```python
from build123d import *

# Parameters (mm, degrees)
SKETCH1_W           = 45
SKETCH1_H           = 45
SKETCH1_R           = 2.6
BOSS_EXTRUDE1_DEPTH = 7.5
SKETCH2_R           = 8.1
CUT_EXTRUDE1_DEPTH  = 6
CUT_EXTRUDE4_START  = -6
SKETCH5_R           = 8.1
CUT_EXTRUDE4_DEPTH  = 6
SKETCH7_W           = 37
SKETCH7_H           = 7
BOSS_EXTRUDE2_DEPTH = 10
CUT_EXTRUDE6_START  = 2
CUT_EXTRUDE6_DEPTH  = 3.6
SKETCH8_R           = 2.1
CUT_EXTRUDE7_DEPTH  = 43.278836313
SKETCH9_W           = 3
SKETCH9_H           = 7
BOSS_EXTRUDE3_DEPTH = 10
SKETCH10_W          = 7
SKETCH10_H          = 7
BOSS_EXTRUDE4_DEPTH = 2
CHAMFER2_SIZE2      = 7
CHAMFER2_SIZE       = 2
CHAMFER3_SIZE2      = 7
CHAMFER3_SIZE       = 2


with BuildPart() as part:
    # Sketch1 → Boss-Extrude1 (new, symmetric)
    with BuildSketch(Plane.XY):
        Rectangle(SKETCH1_W, SKETCH1_H)
        Circle(SKETCH1_R, mode=Mode.SUBTRACT)
    extrude(amount=BOSS_EXTRUDE1_DEPTH, both=True)

    # Sketch2 → Cut-Extrude1 (cut)
    with BuildSketch(Plane.XY.offset(7.5)):
        Circle(SKETCH2_R)
    extrude(amount=-CUT_EXTRUDE1_DEPTH, mode=Mode.SUBTRACT)

    # Sketch5 → Cut-Extrude4 (cut)
    with BuildSketch(Plane(origin=(0, 0, -7.5), x_dir=(-1, 0, 0), z_dir=(0, 0, -1)).offset(CUT_EXTRUDE4_START)):
        with Locations(Location((0, 0, 0), (0, 0, 180))):
            Circle(SKETCH5_R)
    extrude(amount=CUT_EXTRUDE4_DEPTH, mode=Mode.SUBTRACT)

    # Sketch7 → Boss-Extrude2 (add)
    with BuildSketch(Plane.XZ.offset(22.5)):
        Rectangle(SKETCH7_W, SKETCH7_H)
    extrude(amount=BOSS_EXTRUDE2_DEPTH)

    # Sketch6 → Cut-Extrude6 (cut)
    with BuildSketch(Plane.XY.offset(-7.5).offset(CUT_EXTRUDE6_START)):
        Polygon((19.2, 17.636195996), (15.5, 19.772391992), (11.8, 17.636195996), (11.8, 13.363804004), (15.5, 11.227608008), (19.2, 13.363804004), align=None)
        Polygon((-11.8, 17.636195996), (-15.5, 19.772391992), (-19.2, 17.636195996), (-19.2, 13.363804004), (-15.5, 11.227608008), (-11.8, 13.363804004), align=None)
        Polygon((19.2, -13.363804004), (15.5, -11.227608008), (11.8, -13.363804004), (11.8, -17.636195996), (15.5, -19.772391992), (19.2, -17.636195996), align=None)
        Polygon((-11.8, -13.363804004), (-15.5, -11.227608008), (-19.2, -13.363804004), (-19.2, -17.636195996), (-15.5, -19.772391992), (-11.8, -17.636195996), align=None)
    extrude(amount=CUT_EXTRUDE6_DEPTH, mode=Mode.SUBTRACT)

    # Sketch8 → Cut-Extrude7 (cut, through all)
    with BuildSketch(Plane(origin=(0, 0, -7.5), x_dir=(-1, 0, 0), z_dir=(0, 0, -1))):
        with Locations((-15.5, 15.5)):
            Circle(SKETCH8_R)
        with Locations((15.5, 15.5)):
            Circle(SKETCH8_R)
        with Locations((15.5, -15.5)):
            Circle(SKETCH8_R)
        with Locations((-15.5, -15.5)):
            Circle(SKETCH8_R)
    extrude(amount=-CUT_EXTRUDE7_DEPTH, mode=Mode.SUBTRACT)

    # Sketch9 → Boss-Extrude3 (add)
    with BuildSketch(Plane.XZ.offset(32.5)):
        with Locations((-17, 0)):
            Rectangle(SKETCH9_W, SKETCH9_H)
        with Locations((17, 0)):
            Rectangle(SKETCH9_W, SKETCH9_H)
    extrude(amount=BOSS_EXTRUDE3_DEPTH)

    # Sketch10 → Boss-Extrude4 (add)
    with BuildSketch(Plane.ZY.offset(18.5)):
        with Locations((0, -39)):
            Rectangle(SKETCH10_W, SKETCH10_H)
    boss_extrude4 = extrude(amount=BOSS_EXTRUDE4_DEPTH)

    # Mirror1: Boss-Extrude4 across plane
    add(boss_extrude4.mirror(Plane(origin=(0, 0, 0), x_dir=(0, 0, 1), z_dir=(1, 0, 0))))

    # Chamfer2
    chamfer2_edges = [part.edges().sort_by_distance(p)[0] for p in [
        (-20.5, -42.5, 0),
    ]]
    chamfer2_side = [part.faces().sort_by_distance(p)[0] for p in [
        (-20.46, -42.5, 0),
    ]]
    chamfer(chamfer2_edges, length=CHAMFER2_SIZE - 0.0001, length2=CHAMFER2_SIZE2 - 0.0001, reference=chamfer2_side[0])  # a hair under: the kernel refuses the full size

    # Chamfer3
    chamfer3_edges = [part.edges().sort_by_distance(p)[0] for p in [
        (20.5, -42.5, 0),
    ]]
    chamfer3_side = [part.faces().sort_by_distance(p)[0] for p in [
        (20.46, -42.5, 0),
    ]]
    chamfer(chamfer3_edges, length=CHAMFER3_SIZE - 0.0001, length2=CHAMFER3_SIZE2 - 0.0001, reference=chamfer3_side[0])  # a hair under: the kernel refuses the full size


solid = part.part
```
Geometry: final body of the model. Coordinates: model frame, mm. A direction names the side the tool comes from. Round coordinates to 2 decimals unless told otherwise and drop trailing zeros. Order: outer loops, then holes, each group sorted by start corner. A loop starts at its lowest first (then second) coordinate and runs counter-clockwise, first axis right, second up. Notation, with made-up numbers: (49.25, 31) -> (77.25, 31) arc R12 ccw to (77.25, 53) -> close; hole circle Ø2 at (43.5, 18.25). An arc over 180 degrees is marked (long way). Write each question's results on one line, items separated by ' | '.
Q1. Section query C-C (z = 0.75). Count the separate pieces of the cut face and the enclosed holes in it, and give its area (3 significant figures).
Response values:
separate pieces: 1 | enclosed holes: 5 | area: 2,390 mm²
Q2. Pin query (flat end, axial travel): pin 1 Ø8 at (x, y) = (0, -0.5) entering from +Z; pin 2 Ø3 at (y, z) = (-25, -2.5) entering from +X; pin 3 Ø3 at (x, y) = (0, 0) entering from -Z; pin 4 Ø7.5 at (y, z) = (-28.5, -1.5) entering from -X. Return the tip coordinate at first contact, or that it passes through.
Response values:
pin 1: z = 1.5 | pin 2: x = 18.5 | pin 3: through | pin 4: x = -18.5
Q3. Access query for faces 4 (the face through (-1.756, -7.907, 4.542)), 5 (the face through (0, -32.5, 0)), 6 (the face through (13.68, -12.28, -3.73)). Directions: +Z, -Z, +X, -X, +Y, -Y. A direction counts if a zero-diameter tool reaches every point of the face in a straight line with its end or side. Return the directions, or none.
Response values:
face 4: +Z | face 5: +Z, -Z, -Y | face 6: none
Q4. Ray query, line 1 along X through (y, z) = (17.5, -3); line 2 along Z through (x, y) = (18.5, -14.5). Return the intervals inside material, ascending.
Response values:
line 1: -22.5 to -19.2, -11.8 to 11.8, 19.2 to 22.5 | line 2: -7.5 to -5.5, -1.9 to 7.5
Q5. Pull-direction query (Z, two-part tool) for faces 1 (the face through (0, 10, 7.5)), 2 (the face through (17.376, -12.311, -3.725)), 3 (the face through (-15.227, -13.418, 2.734)); classes: released by +Z, released by -Z, zero draft, split by the parting line, or undercut.
Response values:
face 1: released by +Z | face 2: undercut | face 3: zero draft
Q6. Section query D-D (y = 0). Output: boundary loops of the cut face in (x, z).
Response values:
outline: (-22.5, -7.5) -> (-8.1, -7.5) -> (-8.1, -1.5) -> (-2.6, -1.5) -> (-2.6, 1.5) -> (-8.1, 1.5) -> (-8.1, 7.5) -> (-22.5, 7.5) -> close; (2.6, -1.5) -> (8.1, -1.5) -> (8.1, -7.5) -> (22.5, -7.5) -> (22.5, 7.5) -> (8.1, 7.5) -> (8.1, 1.5) -> (2.6, 1.5) -> close
Q7. Section query A-A (x = 0). Output: boundary loops of the cut face in (y, z), and give its area (3 significant figures).
Response values:
outline: (-32.5, -3.5) -> (-22.5, -3.5) -> (-22.5, -7.5) -> (-8.1, -7.5) -> (-8.1, -1.5) -> (-2.6, -1.5) -> (-2.6, 1.5) -> (-8.1, 1.5) -> (-8.1, 7.5) -> (-22.5, 7.5) -> (-22.5, 3.5) -> (-32.5, 3.5) -> close; (2.6, -1.5) -> (8.1, -1.5) -> (8.1, -7.5) -> (22.5, -7.5) -> (22.5, 7.5) -> (8.1, 7.5) -> (8.1, 1.5) -> (2.6, 1.5) -> close | area: 535 mm²
Q8. Section query B-B (y = -15.5). Output: boundary loops of the cut face in (x, z).
Response values:
outline: (-22.5, -7.5) -> (-17.6, -7.5) -> (-17.6, -5.5) -> (-19.2, -5.5) -> (-19.2, -1.9) -> (-17.6, -1.9) -> (-17.6, 7.5) -> (-22.5, 7.5) -> close; (-13.4, -7.5) -> (13.4, -7.5) -> (13.4, -5.5) -> (11.8, -5.5) -> (11.8, -1.9) -> (13.4, -1.9) -> (13.4, 7.5) -> (-13.4, 7.5) -> (-13.4, -1.9) -> (-11.8, -1.9) -> (-11.8, -5.5) -> (-13.4, -5.5) -> close; (17.6, -7.5) -> (22.5, -7.5) -> (22.5, 7.5) -> (17.6, 7.5) -> (17.6, -1.9) -> (19.2, -1.9) -> (19.2, -5.5) -> (17.6, -5.5) -> close
